from build123d import *

# Parameters (mm, degrees)
SKETCH_1_W        = 28
SKETCH_1_H        = 26
EXTRUDE_1_DEPTH   = 5
EXTRUDE_1_2_DEPTH = 5
EXTRUDE_START     = 10
SKETCH_1_12_W     = 50
SKETCH_1_12_H     = 100
EXTRUDE_2_DEPTH   = 5
SKETCH_2_W        = 40
SKETCH_2_H        = 5
EXTRUDE_3_DEPTH   = 5


with BuildPart() as part:
    # 草图1 → 凸台-拉伸1 (new body)
    with BuildSketch(Plane(origin=(0, 0, 0), x_dir=(1, 0, 0), z_dir=(0, 1, 0))):
        with Locations((106, 29.5)):
            Rectangle(SKETCH_1_W, SKETCH_1_H)
    extrude(amount=EXTRUDE_1_DEPTH)


with BuildPart() as body_2:
    # 草图1 → Extrude 1 2 (new body)
    with BuildSketch(Plane(origin=(0, 0, 0), x_dir=(1, 0, 0), z_dir=(0, 1, 0))):
        with Locations((106, -29.5)):
            Rectangle(SKETCH_1_W, SKETCH_1_H)
    extrude(amount=EXTRUDE_1_2_DEPTH)


with BuildPart() as body_3:
    # 草图1<12> → 凸台-拉伸2 (new body)
    with BuildSketch(Plane(origin=(0, 0, 0), x_dir=(1, 0, 0), z_dir=(0, 1, 0)).offset(EXTRUDE_START)):
        with Locations((25, 0)):
            Rectangle(SKETCH_1_12_W, SKETCH_1_12_H)
    extrude(amount=EXTRUDE_2_DEPTH)

    # 草图2 → 凸台-拉伸3 (add)
    with BuildSketch(Plane(origin=(50, 0, 0), x_dir=(0, 0, -1), z_dir=(1, 0, 0))):
        with Locations((30, 12.5)):
            Rectangle(SKETCH_2_W, SKETCH_2_H)
        with Locations((-30, 12.5)):
            Rectangle(SKETCH_2_W, SKETCH_2_H)
    extrude(amount=EXTRUDE_3_DEPTH)


    add(body_2.part)  # loft_5 joins it to this body
    # loft from a face of the part (loft_5)
    loft([body_3.faces().sort_by_distance((55, 12.5, 30))[0], body_3.faces().sort_by_distance((92, 2.5, 29.5))[0]])


    add(part.part)  # loft_6 joins it to this body
    # loft from a face of the part (loft_6)
    loft([body_3.faces().sort_by_distance((55, 12.5, -30))[0], body_3.faces().sort_by_distance((92, 2.5, -29.5))[0]])


solid = body_3.part
Check sheet for the modelled part. Datum: model origin and axes. Units: mm. A direction names the side the tool comes from. Round coordinates to 2 decimals unless told otherwise and drop trailing zeros. Order: outer loops, then holes, each group sorted by start corner. A loop starts at its lowest first (then second) coordinate and runs counter-clockwise, first axis right, second up.
Q1. Set-up check for faces 1 (the face through (106, 2, -42.5)), 2 (the face through (106, 5, 29)), 3 (the face through (52, 12, -10)): record each of +Z, -Z, +X, -X, +Y, -Y from which the full face is reachable in a straight line by a thin tool's end or side.
Filled sheet:
face 1: -Z, +X, +Y, -Y
face 2: +Z, -Z, +X, +Y
face 3: +X, +Y, -Y
Q2. Depth check by flat-ended pin: P1, Ø21, axis at x = 103.5, z = -30, coming from the +Y side; P2, Ø2.5, axis at x = 106.5, y = 1.5, coming from the -Z side; P3, Ø4, axis at y = 12.5, z = -3, coming from the +X side. Enter the tip coordinate at first touch or a pass-through.
Filled sheet:
P1: stops at y = 5
P2: stops at z = -42.5
P3: stops at x = 50
Q3. Draft check along Z on faces 4 (the face through (106, 0, 29)), 5 (the face through (106, 2, -16.5)), 6 (the face through (27, 12, 50)). Enter one of: pulls with the +Z half, pulls with the -Z half, needs draft (parallel to the pull), parting line crosses it, or undercut.
Filled sheet:
face 4: needs draft
face 5: undercut
face 6: pulls with the +Z half
Q4. Cross-section at C-C, the plane z = 0. Enter the section's corners in (x, y), plus the area to 3 significant figures.
Filled sheet:
outline: (0, 10) - (50, 10) - (50, 15) - (0, 15) - close
area: 250 mm2
Q5. Cross-section at B-B, the plane x = 13.5. Enter the section's corners in (y, z).
Filled sheet:
outline: (10, -50) - (15, -50) - (15, 50) - (10, 50) - close
Q6. Scan lines: L1, parallel to Z at x = 101.5, y = 3.25; L2, parallel to Z at x = 64.5, y = 7.5; L3, parallel to Y at x = 27, z = -28.5. Record each from-to range of solid material in increasing order.
Filled sheet:
L1: z = -42.5 to -16.5, 16.5 to 42.5
L2: z = -48.07 to -11.67, 11.67 to 48.07
L3: y = 10 to 15
Q7. Cross-section at A-A, the plane x = 112. Enter the section's corners in (y, z), plus the area to 3 significant figures.
Filled sheet:
outline: (0, -42.5) - (5, -42.5) - (5, -16.5) - (0, -16.5) - close; (0, 16.5) - (5, 16.5) - (5, 42.5) - (0, 42.5) - close
area: 260 mm2
